The figure shows three views and two pictorial views of one solid part (mm, origin at its lowest corner). Answer the questions. A direction names the side the tool comes from. Give positions to 0.01 mm unless a question says otherwise; leave off trailing zeros. Order: outer loops, then holes, each group sorted by start corner. A loop starts at its lowest first (then second) coordinate and runs counter-clockwise, first axis right, second up. Notation, with made-up numbers: (20, -21.75) -> (24, -21.75) arc R18 cw to (24, 11.25) -> close; hole circle Ø11 at (-26.75, 48). An arc over 180 degrees is marked (long way). Use one line per item in the form item = value.
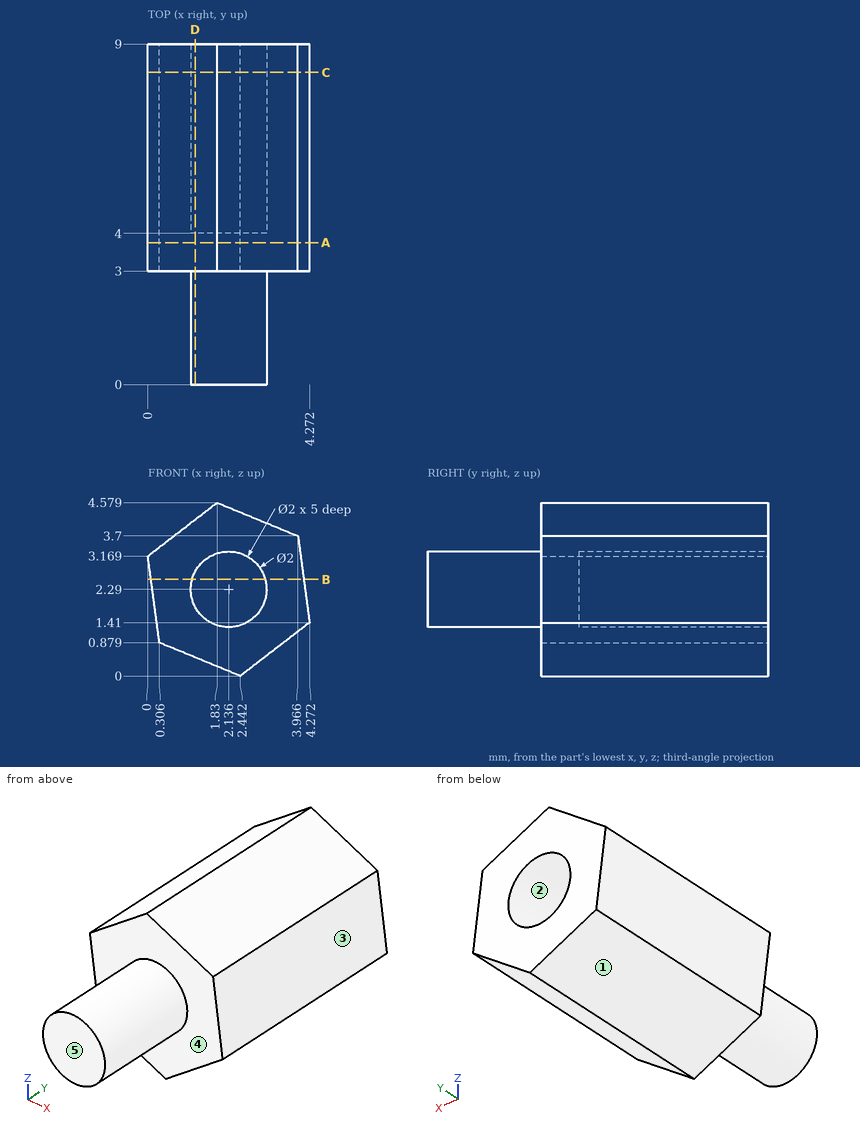
Item 1: Straight lines are drawn through the part: L1, parallel to Y at x = 3.2, z = 2.2; L2, parallel to X at y = 5, z = 2.3 (1 decimal); L3, parallel to Z at x = 1.5, y = 5.25 (1 decimal). For each, find the intervals that lie inside material, in ascending order. Write a range as from..to.
Checks:
L1 = 3..9
L2 = 0.1..1.1, 3.1..4.2
L3 = 0.4..1.5, 3.1..4.3
Item 2: The part is cut by section A-A on y = 3.75. Give the vertices of the cut face in (x, z) (1 decimal).
Checks:
outline = (0, 3.2) -> (0.3, 0.9) -> (2.4, 0) -> (4.3, 1.4) -> (4, 3.7) -> (1.8, 4.6) -> close
Item 3: Determine the mould class of the marked faces 1, 2 and 3 for opening direction Z: +Z half, -Z half, draft (parallel to the pull), parting line (faces both ways), or undercut.
Checks:
face_1 = -Z half
face_2 = undercut
face_3 = +Z half
Item 4: Which of the six approach directions +Z, -Z, +X, -X, +Y, -Y give full straight-line access (tool end or side, diameter ignored) to the marked faces 4 and 5?
Checks:
face_4 = -Y
face_5 = +Z, -Z, +X, -X, -Y
Item 5: The part is cut by section D-D on x = 1.25. Give the vertices of the cut face in (y, z).
Checks:
outline = (0, 1.83) -> (3, 1.83) -> (3, 0.49) -> (9, 0.49) -> (9, 1.83) -> (4, 1.83) -> (4, 2.75) -> (9, 2.75) -> (9, 4.13) -> (3, 4.13) -> (3, 2.75) -> (0, 2.75) -> close
Item 6: The part is cut by section B-B on z = 2.55. Give the vertices of the cut face in (x, y).
Checks:
outline = (0.08, 3) -> (1.17, 3) -> (1.17, 0) -> (3.1, 0) -> (3.1, 3) -> (4.12, 3) -> (4.12, 9) -> (3.1, 9) -> (3.1, 4) -> (1.17, 4) -> (1.17, 9) -> (0.08, 9) -> close
Item 7: The part is cut by section C-C on y = 8.25. Give the vertices of the cut face in (x, z) (1 decimal).
Checks:
outline = (0, 3.2) -> (0.3, 0.9) -> (2.4, 0) -> (4.3, 1.4) -> (4, 3.7) -> (1.8, 4.6) -> close; hole circle Ø2 at (2.1, 2.3)
